from build123d import *

# Parameters (mm, degrees)
CROQUIS1_W              = 50
CROQUIS1_H              = 110
SALIENTE_EXTRUIR1_DEPTH = 1.5
CROQUIS2_R              = 2.5
SALIENTE_EXTRUIR2_DEPTH = 5
CHAFL_N1_SIZE           = 1.3
REDONDEO1_R             = 1
CORTAR_EXTRUIR1_DEPTH   = 10


with BuildPart() as part:
    # Croquis1 → Saliente-Extruir1 (new body)
    with BuildSketch(Plane.XY):
        Rectangle(CROQUIS1_W, CROQUIS1_H)
    extrude(amount=SALIENTE_EXTRUIR1_DEPTH)

    # Croquis2 → Saliente-Extruir2 (add)
    with BuildSketch(Plane.XY.offset(1.5)):
        with Locations((-15, 50)):
            Circle(CROQUIS2_R)
        with Locations((-21, 45)):
            Circle(CROQUIS2_R)
        with Locations((-15, 40)):
            Circle(CROQUIS2_R)
        with Locations((-9, 45)):
            Circle(CROQUIS2_R)
        with Locations((-15, -40)):
            Circle(CROQUIS2_R)
        with Locations((-9, -45)):
            Circle(CROQUIS2_R)
        with Locations((-15, -50)):
            Circle(CROQUIS2_R)
        with Locations((-21, -45)):
            Circle(CROQUIS2_R)
        with Locations(Location((21, -45, 0), (0, 0, 180))):
            Circle(CROQUIS2_R)
        with Locations(Location((15, -50, 0), (0, 0, 180))):
            Circle(CROQUIS2_R)
        with Locations(Location((9, -45, 0), (0, 0, 180))):
            Circle(CROQUIS2_R)
        with Locations(Location((15, -40, 0), (0, 0, 180))):
            Circle(CROQUIS2_R)
        with Locations(Location((21, 45, 0), (0, 0, 180))):
            Circle(CROQUIS2_R)
        with Locations(Location((15, 50, 0), (0, 0, 180))):
            Circle(CROQUIS2_R)
        with Locations(Location((9, 45, 0), (0, 0, 180))):
            Circle(CROQUIS2_R)
        with Locations(Location((15, 40, 0), (0, 0, 180))):
            Circle(CROQUIS2_R)
    extrude(amount=SALIENTE_EXTRUIR2_DEPTH)

    # Chafl_n1
    chafl_n1_edges = [part.edges().sort_by_distance(p)[0] for p in [
        (-17.5, 50, 6.5),
        (-23.5, 45, 6.5),
        (-17.5, 40, 6.5),
        (-11.5, 45, 6.5),
        (-17.5, -40, 6.5),
        (-11.5, -45, 6.5),
        (-17.5, -50, 6.5),
        (-23.5, -45, 6.5),
        (23.5, -45, 6.5),
        (17.5, -50, 6.5),
        (11.5, -45, 6.5),
        (17.5, -40, 6.5),
        (23.5, 45, 6.5),
        (17.5, 50, 6.5),
        (11.5, 45, 6.5),
        (17.5, 40, 6.5),
    ]]
    chamfer(chafl_n1_edges, length=CHAFL_N1_SIZE)

    # Redondeo1
    redondeo1_edges = [part.edges().sort_by_distance(p)[0] for p in [
        (0, -55, 0),
        (-25, 0, 0),
        (0, 55, 0),
        (25, 0, 0),
    ]]
    fillet(redondeo1_edges, radius=REDONDEO1_R)

    # Croquis3 → Cortar-Extruir1 (cut)
    with BuildSketch(Plane(origin=(0, 0, 0), x_dir=(-1, 0, 0), z_dir=(0, 0, -1))):
        with BuildLine():
            add(Edge.make_bspline(
                [(22.361475253, -39.186991388), (10.271319675, 11.528482347), (23.288602916, 40.714890738)],
                knots=[0, 0, 0, 1, 1, 1], degree=2))
            add(Edge.make_bspline(
                [(22.361475253, -39.186991388), (20.200722134, -14.449114626), (20.113642926, 12.226208442), (23.288602916, 40.714890738)],
                knots=[0, 0, 0, 0, 1, 1, 1, 1], degree=3))
        make_face()
        with BuildLine():
            add(Edge.make_bspline(
                [(-22.361475253, -39.186991388), (-20.200722134, -14.449114626), (-20.113642926, 12.226208442), (-23.288602916, 40.714890738)],
                knots=[0, 0, 0, 0, 1, 1, 1, 1], degree=3))
            add(Edge.make_bspline(
                [(-22.361475253, -39.186991388), (-10.271319675, 11.528482347), (-23.288602916, 40.714890738)],
                knots=[0, 0, 0, 1, 1, 1], degree=2))
        make_face()
    extrude(amount=-CORTAR_EXTRUIR1_DEPTH, mode=Mode.SUBTRACT)


solid = part.part
Model file for the job. Use its own axes, mm. A direction names the side the tool comes from. Coordinates: 2 decimals unless noted, no trailing zeros. Order: outer loops, then holes, each group sorted by start corner. A loop starts at its lowest first (then second) coordinate and runs counter-clockwise, first axis right, second up. Notation, with made-up numbers: M 0,55.5 L 47,55.5 A20 cw 47,73.5 Z; hole C -20,43.25 d8. An arc over 180 degrees is marked long. Return JSON: item names as keys, results as strings.
1. Tool access for faces 1 (the face through (15.54, 42.44, 3.32)), 2 (the face through (-15, -40, 6.5)): list every direction of +Z, -Z, +X, -X, +Y, -Y with a clear straight run to the whole face (end or side of a thin tool).
Ans:
{"face 1": "+Z", "face 2": "+Z, +X, -X, +Y, -Y"}
2. Flat gauge pin, fed straight in: pin 1 (3 mm diameter, centred on x = 16.5, z = 5.5, fed in from +Y). Where does the tip first touch, or does it go through?
Ans:
{"pin 1": "y = 52.5"}
3. Saw through at A-A (z = 3.75). Give the number of separate pieces and of enclosed holes in the cut face, and give its area (3 significant figures).
Ans:
{"separate pieces": "16", "enclosed holes": "0", "area": "314 mm^2"}
4. Saw through at C-C (y = 50). Give the cut face in (x, z).
Ans:
{"outline": "M -25,1 A1 ccw -24,0 L 24,0 A1 ccw 25,1 L 25,1.5 L 17.5,1.5 L 17.5,5.2 L 16.2,6.5 L 13.8,6.5 L 12.5,5.2 L 12.5,1.5 L -12.5,1.5 L -12.5,5.2 L -13.8,6.5 L -16.2,6.5 L -17.5,5.2 L -17.5,1.5 L -25,1.5 Z"}
5. Pull direction Y, two halves, no side cores. Call faces 3 (the face through (-23, -46.5, 3.3)), 4 (the face through (15.54, 52.44, 3.32)), 5 (the face through (21, 45, 6.5)): +Y half, -Y half, draft (parallel to the pull), parting line (faces both ways), or undercut.
Ans:
{"face 3": "undercut", "face 4": "undercut", "face 5": "draft"}
6. Saw through at D-D (x = 9). Give the cut face in (y, z).
Ans:
{"outline": "M -55,1 A1 ccw -54,0 L 54,0 A1 ccw 55,1 L 55,1.5 L 47.5,1.5 L 47.5,5.2 L 46.2,6.5 L 43.8,6.5 L 42.5,5.2 L 42.5,1.5 L -42.5,1.5 L -42.5,5.2 L -43.8,6.5 L -46.2,6.5 L -47.5,5.2 L -47.5,1.5 L -55,1.5 Z"}
7. Drill centre lines: probe 1 along Y at (x, z) = (14, 3); probe 2 along Y at (x, z) = (-17, 5.25); probe 3 along Z at (x, y) = (-10.5, -48.5). Where is each one in solid material? Low to high.
Ans:
{"probe 1": "-52.29 to -47.71, -42.29 to -37.71, 37.71 to 42.29, 47.71 to 52.29", "probe 2": "-51.42 to -48.58, -41.42 to -38.58, 38.58 to 41.42, 48.58 to 51.42", "probe 3": "0 to 1.5"}
